Source: CAD feature listing. Evaluate the final solid. Frame: model axes, mm. A direction names the side the tool comes from. Coordinates: 2 decimals unless noted, no trailing zeros. Loops run counter-clockwise (first coordinate to the right, second up) from the corner with the lowest first, then second, coordinate; pieces in that order, holes last. Notation, with made-up numbers: M 68.5,-21 L 118.5,-21 A9 ccw 118.5,-10 Z; hole C 81,-3.75 d6. An arc over 180 degrees is marked long. Write each question's results on one line, items separated by ' | '. Start each with the question number.
from build123d import *

# Parameters (mm, degrees)
F1_DEPTH = 25
F2_F1_R  = 5
F2_F2_R  = 5


with BuildPart() as f1:
    # F0 (on Top) → F1 (new body)
    with BuildSketch(Plane.XY):
        Polygon((0, 50.3999988563), (-80, 50.3999988563), (-80, 26.3999988563), (-40, 26.3999988563), (-40, 2.3999988563), (40, 2.3999988563), (40, 26.3999988563), (80, 26.3999988563), (80, 50.3999988563), align=None)
    extrude(amount=F1_DEPTH)

    # F2: fillet of radius 5 on 23 edges, made by hand

    # F2_f1
    f2_f1_edges = [f1.edges().sort_by_distance(p)[0] for p in [
        (40, 26.3999988563, 12.5),
        (-40, 26.3999988563, 12.5),
    ]]
    fillet(f2_f1_edges, radius=F2_F1_R)

    # F2_f2
    f2_f2_edges = [f1.edges().sort_by_distance(p)[0] for p in [
        (0, 2.3999988563, 25),
        (-40, 11.8999988563, 25),
        (0, 50.3999988563, 25),
        (-80, 38.3999988563, 25),
        (-62.5, 26.3999988563, 25),
        (40, 11.8999988563, 25),
        (62.5, 26.3999988563, 25),
        (80, 38.3999988563, 25),
        (40, 2.3999988563, 12.5),
        (0, 2.3999988563, 0),
        (40, 11.8999988563, 0),
        (62.5, 26.3999988563, 0),
        (80, 26.3999988563, 12.5),
        (80, 38.3999988563, 0),
        (80, 50.3999988563, 12.5),
        (-40, 2.3999988563, 12.5),
        (-80, 26.3999988563, 12.5),
        (-62.5, 26.3999988563, 0),
        (-80, 50.3999988563, 12.5),
        (-80, 38.3999988563, 0),
        (0, 50.3999988563, 0),
        (-41.4644660941, 24.9355327622, 0),
        (41.4644660941, 24.9355327622, 0),
        (41.4644660941, 24.9355327622, 25),
        (-41.4644660941, 24.9355327622, 25),
    ]]
    fillet(f2_f2_edges, radius=F2_F2_R)


solid = f1.part
Item 1: Cut plane A-A (z = 14). Output: boundary loops of the cut face in (x, y), then the cut area to 3 significant figures.
Item 2: Line query: probe 1 along Y at (x, z) = (-44.5, 8); probe 2 along X at (y, z) = (10, 9); probe 3 along Y at (x, z) = (-65.5, 24). Output: solid intervals per line, ascending.
Item 3: Access query for faces 1 (the cylindrical face through (60.21, 27.9, 23.57)), 2 (the flat face through (40, 14, 12)), 3 (the cylindrical face through (-59.79, 27.9, 23.57)), 4 (the flat face through (-40, 14, 12)), 5 (the cylindrical face through (60.21, 27.9, 1.43)). Directions: +Z, -Z, +X, -X, +Y, -Y. A direction counts if a zero-diameter tool reaches every point of the face in a straight line with its end or side. Return the directions, or none.
Item 4: Cut plane D-D (z = 2.25). Output: boundary loops of the cut face in (x, y).
Item 5: Cut plane B-B (x = 18). Output: boundary loops of the cut face in (y, z), then the cut area to 3 significant figures.
Item 6: Cut plane C-C (y = 12.5). Output: boundary loops of the cut face in (x, z), then the cut area to 3 significant figures.
Item 7: First-contact query: pin 1 Ø1.5 at (y, z) = (30.5, 12.5) entering from -X; pin 2 Ø4.5 at (x, z) = (60.5, 16) entering from -Y; pin 3 Ø4 at (y, z) = (15, 13) entering from -X. Flat tips, straight axial feed; report the tip coordinate or a pass-through.
Response values:
1) outline: M -80,31.4 A5 ccw -75,26.4 L -45,26.4 A5 cw -40,21.4 L -40,7.4 A5 ccw -35,2.4 L 35,2.4 A5 ccw 40,7.4 L 40,21.4 A5 cw 45,26.4 L 75,26.4 A5 ccw 80,31.4 L 80,45.4 A5 ccw 75,50.4 L -75,50.4 A5 ccw -80,45.4 Z | area: 5,740 mm2
2) probe 1: y = 26.37 to 50.4 | probe 2: x = -40 to 40 | probe 3: y = 28.4 to 48.4
3) face 1: +Z, +X, -Y | face 2: +Z, -Z, +X, -Y | face 3: +Z, -X, -Y | face 4: +Z, -Z, -X, -Y | face 5: -Z, +X, -Y
4) outline: M -79.18,31.4 A4.18 ccw -75,27.22 L -45,27.22 A5.82 cw -39.18,21.4 L -39.18,7.4 A4.18 ccw -35,3.22 L 35,3.22 A4.18 ccw 39.18,7.4 L 39.18,21.4 A5.82 cw 45,27.22 L 75,27.22 A4.18 ccw 79.18,31.4 L 79.18,45.4 A4.18 ccw 75,49.58 L -75,49.58 A4.18 ccw -79.18,45.4 Z
5) outline: M 2.4,5 A5 ccw 7.4,0 L 45.4,0 A5 ccw 50.4,5 L 50.4,20 A5 ccw 45.4,25 L 7.4,25 A5 ccw 2.4,20 Z | area: 1,180 mm2
6) outline: M -40,5 A5 ccw -35,0 L 35,0 A5 ccw 40,5 L 40,20 A5 ccw 35,25 L -35,25 A5 ccw -40,20 Z | area: 1,980 mm2
7) pin 1: stops at x = -80 | pin 2: stops at y = 26.4 | pin 3: stops at x = -40
